```python
from build123d import *

# Parameters (mm, degrees)
SKETCH_W                = 14.6
SKETCH_H                = 5
PAD_DEPTH               = 2.5
SKETCH001_R             = 2.5
SKETCH001_R_2           = 1.8
PAD001_DEPTH            = 2.5
SKETCH002_W             = 0.8
SKETCH002_H             = 1.3
PAD002_DEPTH            = 5.5
SKETCH002_MIRRORED_2_W  = 0.8
SKETCH002_MIRRORED_2_H  = 1.3
PAD002_MIRRORED_2_DEPTH = 5.5
LINEARPATTERN_COUNT     = 4
LINEARPATTERN_PITCH     = 3.2


with BuildPart() as part:
    # Sketch → Pad (new body, symmetric)
    with BuildSketch(Plane.YZ):
        with Locations((-7.3, 2.5)):
            Rectangle(SKETCH_W, SKETCH_H)
    extrude(amount=PAD_DEPTH, both=True)

    # Sketch001 (on Face2 of Pad) → Pad001 (join)
    with BuildSketch(Plane.ZX):
        with Locations((2.5, 0)):
            Circle(SKETCH001_R)
        with Locations((2.5, 0)):
            Circle(SKETCH001_R_2, mode=Mode.SUBTRACT)
    extrude(amount=PAD001_DEPTH)

    # Sketch002 → Pad002 (join)
    with BuildSketch(Plane.XY.offset(2.5)):
        with Locations((-2.85, -11.4)):
            Rectangle(SKETCH002_W, SKETCH002_H)
    pad002 = extrude(amount=-PAD002_DEPTH)

    # Sketch002 Mirrored 2 → Pad002 Mirrored 2 (add)
    with BuildSketch(Plane(origin=(0, 0, 2.5), x_dir=(-1, 0, 0), z_dir=(0, 0, -1))):
        with Locations((-2.85, -11.4)):
            Rectangle(SKETCH002_MIRRORED_2_W, SKETCH002_MIRRORED_2_H)
    pad002_mirrored_2 = extrude(amount=PAD002_MIRRORED_2_DEPTH)

    # LinearPattern: Pad002, Pad002 Mirrored 2 ×4
    with Locations(*[(0, i * LINEARPATTERN_PITCH, 0) for i in range(1, LINEARPATTERN_COUNT)]):
        add(pad002)
        add(pad002_mirrored_2)


solid = part.part
```
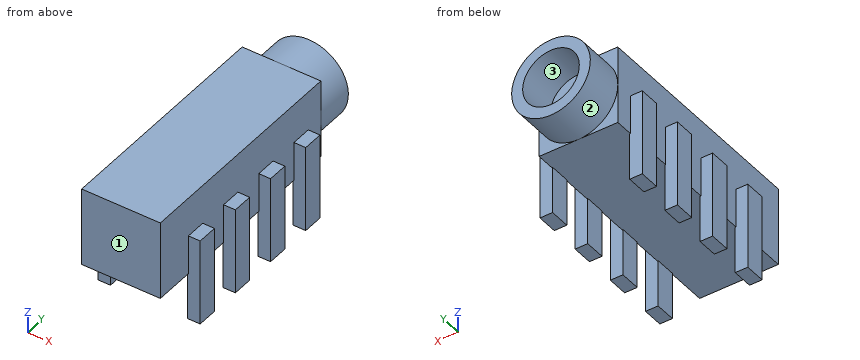
Source: CAD feature listing. Evaluate the final solid. Frame: model axes, mm. Face numbers are marked on the shaded views. Coordinates: 2 decimals unless noted, no trailing zeros. Order: outer loops, then holes, each group sorted by start corner. A loop starts at its lowest first (then second) coordinate and runs counter-clockwise, first axis right, second up. Notation, with made-up numbers: (44, 16.5) - (84, 16.5) arc R29 ccw to (84, 52.5) - close; hole circle Ø4 at (15.25, 80). An arc over 180 degrees is marked (long way). One line per item, written item: value.
1) Ray query, line 1 (X direction, y = 1.05, z = 2.5); line 2 (X direction, y = -12, z = -0.5); line 3 (Z direction, x = 0.5, y = -1.5). Return the intervals inside material, ascending. Write a range as [from, to].
Computed values:
line 1: x = [-2.5, -1.8], [1.8, 2.5]
line 2: x = [-3.25, -2.45], [2.45, 3.25]
line 3: z = [0, 5]
2) Mould query, pull axis Z, two halves, no side actions, for the marked faces 1, 2 and 3. Classes: released by +Z, released by -Z, zero draft, split by the parting line, or undercut.
Computed values:
face 1: zero draft
face 2: split by the parting line
face 3: undercut
3) Cut plane B-B on z = -2. State how many separate pieces and enclosed holes the cut face has, plus the area to 3 significant figures.
Computed values:
separate pieces: 8
enclosed holes: 0
area: 8.32 mm^2
4) Contact query for flat-ended pins moving along their axis: pin 1 (0.9 mm diameter, centred on x = 2.5, z = -1, fed in from -Y); pin 2 (0.6 mm diameter, centred on x = -3, z = 1, fed in from +Y); pin 3 (1 mm diameter, centred on x = 1, y = -4, fed in from -Z). Output: stop coordinate, or through.
Computed values:
pin 1: stops at y = -12.05
pin 2: stops at y = -1.15
pin 3: stops at z = 0
5) Cut plane C-C on y = -11.25. Output: boundary loops of the cut face in (x, z), plus the area to 4 significant figures.
Computed values:
outline: (-3.25, -3) - (-2.45, -3) - (-2.45, 0) - (2.45, 0) - (2.45, -3) - (3.25, -3) - (3.25, 2.5) - (2.5, 2.5) - (2.5, 5) - (-2.5, 5) - (-2.5, 2.5) - (-3.25, 2.5) - close
area: 33.55 mm^2
6) Cut plane D-D on x = 0.75. Output: boundary loops of the cut face in (y, z), plus the area to 3 significant figures.
Computed values:
outline: (-14.6, 0) - (0, 0) - (0, 0.12) - (2.5, 0.12) - (2.5, 0.86) - (0, 0.86) - (0, 4.14) - (2.5, 4.14) - (2.5, 4.88) - (0, 4.88) - (0, 5) - (-14.6, 5) - close
area: 76.7 mm^2
7) Cut plane A-A on x = 2.75. Output: boundary loops of the cut face in (y, z).
Computed values:
outline: (-12.05, -3) - (-10.75, -3) - (-10.75, 2.5) - (-12.05, 2.5) - close; (-8.85, -3) - (-7.55, -3) - (-7.55, 2.5) - (-8.85, 2.5) - close; (-5.65, -3) - (-4.35, -3) - (-4.35, 2.5) - (-5.65, 2.5) - close; (-2.45, -3) - (-1.15, -3) - (-1.15, 2.5) - (-2.45, 2.5) - close
